```python
from build123d import *

# Parameters (mm, degrees)
SKETCH1_W                  = 43
SKETCH1_H                  = 43
BOSS_EXTRUDE1_DEPTH        = 24
SKETCH2_W                  = 38.4
SKETCH2_H                  = 38.2
CUT_EXTRUDE1_DEPTH         = 1.7
F_1_6_1_6_DIAMETER_HOLE1_D = 1.6
SKETCH5_W                  = 30.2
SKETCH5_H                  = 34.1
CUT_EXTRUDE2_DEPTH         = 2
SKETCH6_W                  = 14
SKETCH6_H                  = 12
CUT_EXTRUDE3_DEPTH         = 38.706630717
SKETCH7_W                  = 28.9
SKETCH7_H                  = 55.98263728
CUT_EXTRUDE4_DEPTH         = 37.559403715
SKETCH8_W                  = 7.05
SKETCH8_H                  = 20.3
BOSS_EXTRUDE2_DEPTH        = 8.2
SKETCH9_W                  = 36.19131864
SKETCH9_H                  = 11.8
CUT_EXTRUDE5_DEPTH         = 4.1
F_2_9_2_9_DIAMETER_HOLE1_D = 2.9
SKETCH13_W                 = 45
SKETCH13_H                 = 30.01736272
CUT_EXTRUDE6_DEPTH         = 11.8
SKETCH_1_W                 = 54.379926199
SKETCH_1_H                 = 25.742878229
CUT_EXTRUDE_1_DEPTH        = 61.495371724
SKETCH_2_W                 = 51.169507394
SKETCH_2_H                 = 8.248398276
CUT_EXTRUDE_4_DEPTH        = 10
SKETCH_3_W                 = 38.4
SKETCH_3_H                 = 14
CUT_EXTRUDE_5_DEPTH        = 31.629887365
SKETCH_4_W                 = 43
SKETCH_4_H                 = 3
EXTRUDE_1_DEPTH            = 18
SKETCH_5_R                 = 1.6
CUT_EXTRUDE_6_DEPTH        = 49.463285072
SKETCH_5_4_R               = 2.75
EXTRUDE_2_DEPTH            = 3
FILLET_1_R                 = 1
EXTRUDE_3_DEPTH            = 2.3
EXTRUDE_4_DEPTH            = 2.3
FILLET_2_R                 = 2


with BuildPart() as part:
    # Sketch1 → Boss-Extrude1 (new body)
    with BuildSketch(Plane(origin=(0, 0, 0), x_dir=(1, 0, 0), z_dir=(0, 1, 0))):
        Rectangle(SKETCH1_W, SKETCH1_H)
    extrude(amount=BOSS_EXTRUDE1_DEPTH)

    # Sketch2 → Cut-Extrude1 (cut)
    with BuildSketch(Plane(origin=(0, 24, 0), x_dir=(1, 0, 0), z_dir=(0, 1, 0))):
        with Locations((0, -2.4)):
            Rectangle(SKETCH2_W, SKETCH2_H)
    extrude(amount=-CUT_EXTRUDE1_DEPTH, mode=Mode.SUBTRACT)

    # Ø1.6 (1.6) Diameter Hole1 (through all)
    with Locations(Plane(origin=(-17, 22.3, -14.5), x_dir=(0, 0, 1), z_dir=(0, 1, 0))):
        with Locations((0, 0), (0, 34), (34, 34), (34, 0)):
            Hole(F_1_6_1_6_DIAMETER_HOLE1_D / 2)

    # Sketch5 → Cut-Extrude2 (cut)
    with BuildSketch(Plane(origin=(0, 22.3, 0), x_dir=(1, 0, 0), z_dir=(0, 1, 0))):
        with Locations((0, -4.45)):
            Rectangle(SKETCH5_W, SKETCH5_H)
    extrude(amount=-CUT_EXTRUDE2_DEPTH, mode=Mode.SUBTRACT)

    # Sketch6 → Cut-Extrude3 (cut, through all)
    with BuildSketch(Plane(origin=(0, 22.3, 0), x_dir=(1, 0, 0), z_dir=(0, 1, 0))):
        with Locations((0, 10.7)):
            Rectangle(SKETCH6_W, SKETCH6_H)
    extrude(amount=-CUT_EXTRUDE3_DEPTH, mode=Mode.SUBTRACT)

    # Sketch7 → Cut-Extrude4 (cut, through all)
    with BuildSketch(Plane(origin=(0, 20.3, 0), x_dir=(1, 0, 0), z_dir=(0, 1, 0))):
        with Locations((0, -21.5)):
            Rectangle(SKETCH7_W, SKETCH7_H)
    extrude(amount=-CUT_EXTRUDE4_DEPTH, mode=Mode.SUBTRACT)

    # Sketch8 → Boss-Extrude2 (add)
    with BuildSketch(Plane.XY.offset(21.5)):
        with Locations((-17.975, 10.15)):
            Rectangle(SKETCH8_W, SKETCH8_H)
    boss_extrude2 = extrude(amount=BOSS_EXTRUDE2_DEPTH)

    # Mirror1: Boss-Extrude2 across plane
    add(boss_extrude2.mirror(Plane(origin=(0, 0, 0), x_dir=(0, 0, 1), z_dir=(1, 0, 0))))

    # Sketch9 → Cut-Extrude5 (cut)
    with BuildSketch(Plane(origin=(-14.45, 0, 0), x_dir=(0, 0, -1), z_dir=(1, 0, 0))):
        with Locations((-11.60434068, 5.9)):
            Rectangle(SKETCH9_W, SKETCH9_H)
    cut_extrude5 = extrude(amount=-CUT_EXTRUDE5_DEPTH, mode=Mode.SUBTRACT)

    # Mirror2: Cut-Extrude5 across plane
    add(cut_extrude5.mirror(Plane(origin=(0, 0, 0), x_dir=(0, 0, 1), z_dir=(1, 0, 0))), mode=Mode.SUBTRACT)

    # Ø2.9 (2.9) Diameter Hole1 (through all)
    with Locations(Plane.ZY.offset(21.5)):
        with Locations((6.7, 5.05), (18.7, 5.05)):
            Hole(F_2_9_2_9_DIAMETER_HOLE1_D / 2)

    # Sketch13 → Cut-Extrude6 (cut)
    with BuildSketch(Plane.XZ):
        with Locations((0, -21.5)):
            Rectangle(SKETCH13_W, SKETCH13_H)
    extrude(amount=-CUT_EXTRUDE6_DEPTH, mode=Mode.SUBTRACT)

    # 草图1 → 切除-拉伸1 (cut, through all)
    with BuildSketch(Plane.XY.offset(29.7)):
        with Locations((-0.875867159, 7.428560885)):
            Rectangle(SKETCH_1_W, SKETCH_1_H)
    extrude(amount=-CUT_EXTRUDE_1_DEPTH, mode=Mode.SUBTRACT)

    # 草图2 → 切除-拉伸4 (cut)
    with BuildSketch(Plane(origin=(0, 24, 0), x_dir=(1, 0, 0), z_dir=(0, 1, 0))):
        with Locations((1.669275501, 22.824199138)):
            Rectangle(SKETCH_2_W, SKETCH_2_H)
    extrude(amount=-CUT_EXTRUDE_4_DEPTH, mode=Mode.SUBTRACT)

    # 草图3 → 切除-拉伸5 (cut, through all)
    with BuildSketch(Plane.XZ.offset(-20.3)):
        with Locations((0, 2.5)):
            Rectangle(SKETCH_3_W, SKETCH_3_H)
    extrude(amount=-CUT_EXTRUDE_5_DEPTH, mode=Mode.SUBTRACT)

    # 草图4 → 凸台-拉伸1 (add)
    with BuildSketch(Plane.XZ.offset(-20.3)):
        with Locations((0, -13.2)):
            Rectangle(SKETCH_4_W, SKETCH_4_H)
    extrude(amount=EXTRUDE_1_DEPTH)

    # 草图5 → 切除-拉伸6 (cut, through all)
    with BuildSketch(Plane(origin=(0, 0, -14.7), x_dir=(-1, 0, 0), z_dir=(0, 0, -1))):
        with Locations((-1.9, 5.3)):
            Circle(SKETCH_5_R)
        with Locations((14.1, 5.3)):
            Circle(SKETCH_5_R)
    cut_extrude_6 = extrude(amount=-CUT_EXTRUDE_6_DEPTH, mode=Mode.SUBTRACT)

    # 草图5<4> → 凸台-拉伸2 (add)
    with BuildSketch(Plane(origin=(0, 0, -14.7), x_dir=(-1, 0, 0), z_dir=(0, 0, -1))):
        with Locations(Location((0, 14.3, 0), (0, 0, 180))):
            Circle(SKETCH_5_4_R)
    extrude(amount=EXTRUDE_2_DEPTH)

    # 圆角1
    fillet_1_edges = [part.edges().sort_by_distance(p)[0] for p in [
        (-2.75, 14.3, -17.7),
    ]]
    fillet(fillet_1_edges, radius=FILLET_1_R)

    # 草图6 → 凸台-拉伸3 (add)
    with BuildSketch(Plane(origin=(21.5, 0, 0), x_dir=(0, 0, -1), z_dir=(1, 0, 0))):
        Polygon((-21.5, 20.3), (11.7, 2.3), (11.7, 20.3), align=None)
        Polygon((-9.672401199, 17.3), (8.7, 7.339059591), (8.7, 17.3), align=None, mode=Mode.SUBTRACT)
    extrude(amount=-EXTRUDE_3_DEPTH)

    # 镜向1: 切除-拉伸6 across plane
    add(cut_extrude_6.mirror(Plane(origin=(0, 0, 0), x_dir=(0, 0, 1), z_dir=(1, 0, 0))), mode=Mode.SUBTRACT)

    # 草图7 → 凸台-拉伸4 (add)
    with BuildSketch(Plane.ZY.offset(21.5)):
        Polygon((-11.7, 2.3), (-11.7, 20.3), (21.5, 20.3), align=None)
        Polygon((-8.7, 17.3), (9.672401199, 17.3), (-8.7, 7.339059591), align=None, mode=Mode.SUBTRACT)
    extrude(amount=-EXTRUDE_4_DEPTH)

    # 圆角2
    fillet_2_edges = [part.edges().sort_by_distance(p)[0] for p in [
        (20.35, 17.3, 9.672401199),
        (20.35, 7.339059591, -8.7),
        (20.35, 17.3, -8.7),
        (-20.35, 7.339059591, -8.7),
        (-20.35, 17.3, 9.672401199),
        (-20.35, 17.3, -8.7),
    ]]
    fillet(fillet_2_edges, radius=FILLET_2_R)


solid = part.part
```
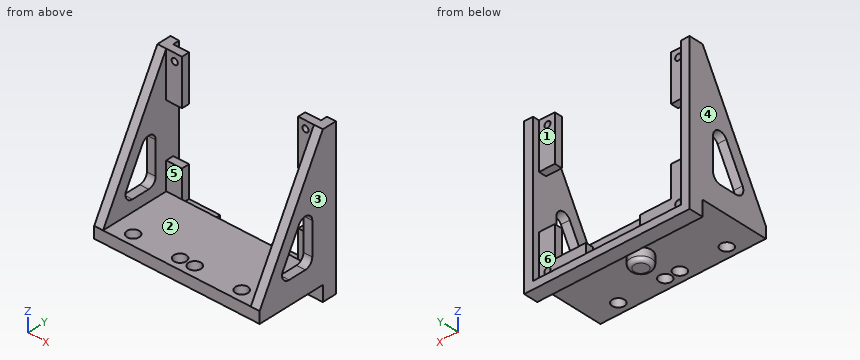
Model file for the job. Use its own axes, mm. Face numbers are marked on the shaded views. A direction names the side the tool comes from. Give positions to 0.01 mm unless a question says otherwise; leave off trailing zeros. Order: outer loops, then holes, each group sorted by start corner. A loop starts at its lowest first (then second) coordinate and runs counter-clockwise, first axis right, second up.
1) Saw through at D-D, the plane x = 17. Write the cut outline in (y, z), then the cut area to 3 significant figures.
2) Saw through at B-B, the plane z = 15.5. Write the cut outline in (x, y), then the cut area to 3 significant figures.
3) Saw through at A-A, the plane x = 4.5. Write the cut outline in (y, z), then the cut area to 3 significant figures.
4) Pin check, flat tips, straight feed: pin 1 (3.5 mm diameter, centred on x = 1.9, y = 5.3, fed in from +Z); pin 2 (2.5 mm diameter, centred on x = 1, z = -13, fed in from +Y); pin 3 (3.5 mm diameter, centred on x = -18, z = -7.5, fed in from -Y); pin 4 (1 mm diameter, centred on x = 17, z = 19.5, fed in from -Y). Stop position of each tip, or through.
5) Wall check: probe 1 along X at (y, z) = (21.2, -14.5); probe 2 along X at (y, z) = (12, 1.5); probe 3 along X at (y, z) = (22.25, 15). Give the ranges that are in metal, low to high.
6) Mould opens along X. For the marked faces 3, 4, 5 and 6 say: +X half, -X half, draft (parallel to the pull), parting line (faces both ways), or undercut.
7) Saw through at C-C, the plane z = -0.5. Write the cut outline in (x, y).
8) 3-axis set-ups, long thin cutter, end or side, ignore diameter. For the marked faces 1 and 2: which of +Z, -Z, +X, -X, +Y, -Y reach the whole face in a straight line?
Computed:
1. outline: (2.3, -14.7) - (20.3, -14.7) - (20.3, -13.7) - (22.3, -13.7) - (22.3, -4.5) - (20.3, -4.5) - (20.3, -11.7) - (2.3, -11.7) - close; (20.3, -18.7) - (24, -18.7) - (24, -16.7) - (22.3, -16.7) - (22.3, -15.3) - (20.3, -15.3) - close; (20.3, 9.5) - (22.3, 9.5) - (22.3, 18.7) - (20.3, 18.7) - close; (20.3, 20.3) - (22.3, 20.3) - (22.3, 21.5) - (20.3, 21.5) - close
1. area: 103 mm2
2. outline: (-21.5, 17.05) - (-19.2, 17.05) - (-19.2, 20.3) - (-15.1, 20.3) - (-15.1, 22.3) - (-19.2, 22.3) - (-19.2, 24) - (-21.5, 24) - close; (15.1, 20.3) - (19.2, 20.3) - (19.2, 17.05) - (21.5, 17.05) - (21.5, 24) - (19.2, 24) - (19.2, 22.3) - (15.1, 22.3) - close
2. area: 48.4 mm2
3. outline: (2.3, -14.7) - (20.3, -14.7) - (20.3, -11.7) - (2.3, -11.7) - close; (20.3, -18.7) - (24, -18.7) - (24, -16.7) - (20.3, -16.7) - close
3. area: 61.4 mm2
4. pin 1: stops at z = -11.7
4. pin 2: stops at y = 20.3
4. pin 3: stops at y = 3.89
4. pin 4: passes through
5. probe 1: x = -21.5 to -17.8, -16.2 to -7, 7 to 16.2, 17.8 to 21.5
5. probe 2: x = -21.5 to -19.2, 19.2 to 21.5
5. probe 3: x = -21.5 to -15.1, 15.1 to 21.5
6. face 3: +X half
6. face 4: -X half
6. face 5: undercut
6. face 6: undercut
7. outline: (-21.5, 8.37) - (-19.2, 8.37) - (-19.2, 11.78) - (-21.5, 11.78) - close; (-21.5, 17.3) - (-19.2, 17.3) - (-19.2, 24) - (-21.5, 24) - close; (19.2, 8.37) - (21.5, 8.37) - (21.5, 11.78) - (19.2, 11.78) - close; (19.2, 17.3) - (21.5, 17.3) - (21.5, 24) - (19.2, 24) - close
8. face 1: +Z, +Y
8. face 2: +Z, -Y
